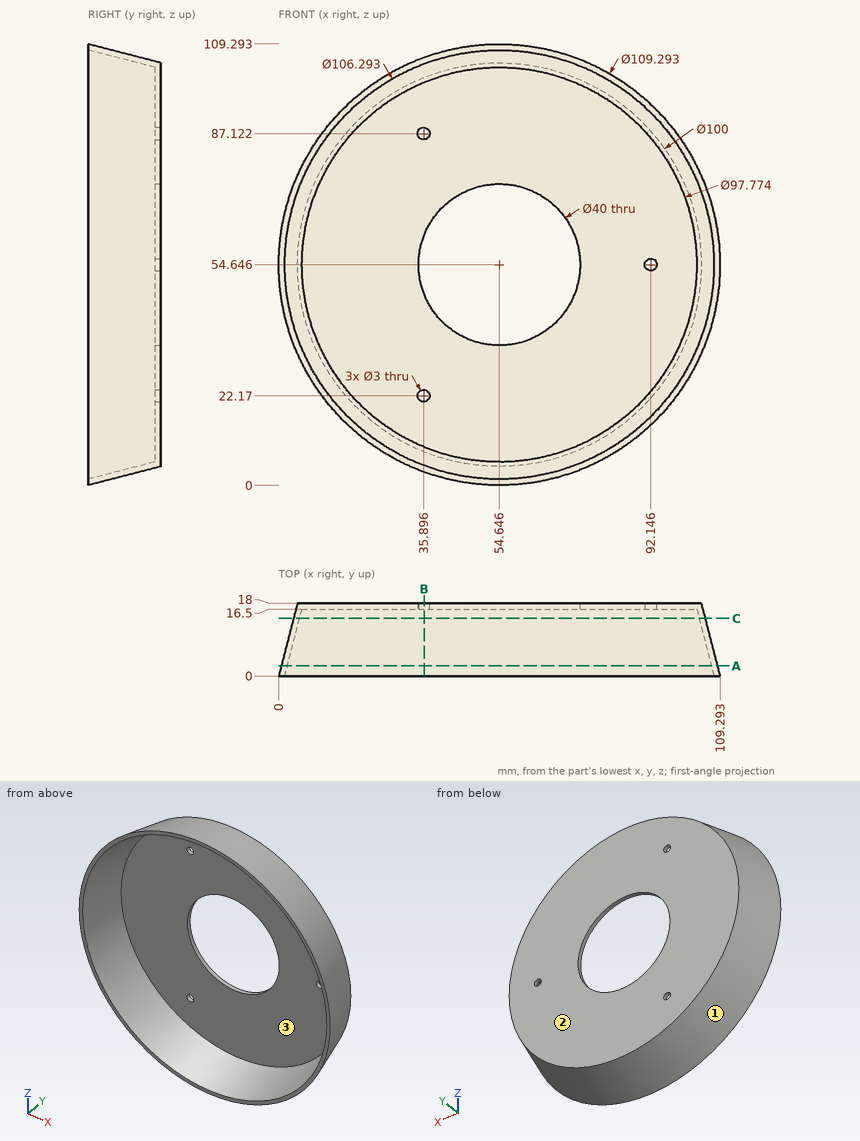
Can you work these out from the drawing? Everything is in mm from the part's minimum corner. Coordinates: 2 decimals unless noted, no trailing zeros. Loops run counter-clockwise (first coordinate to the right, second up) from the corner with the lowest first, then second, coordinate; pieces in that order, holes last.
1) Imagine slicing it at C-C (y = 14.25). List the corners of the cut face in (x, z) for me.
Reported:
outline: circle Ø101.94 at (54.65, 54.65); hole circle Ø98.94 at (54.65, 54.65)
2) Thinking about a two-plate mould opening in X: for the marked faces 1, 2 and 3, which applies, released by +X, released by -X, zero draft, split by the parting line, or undercut?
Reported:
face 1: split by the parting line
face 2: zero draft
face 3: undercut
3) Please list where these lines run through material, in increasing order: line 1 along Y through (x, z) = (29, 71.5); line 2 along X through (y, z) = (3.5, 43.5); line 3 along Z through (x, y) = (55, 8.75).
Reported:
line 1: y = 16.5 to 18
line 2: x = 2.07 to 3.61, 105.69 to 107.22
line 3: z = 2.26 to 3.76, 105.53 to 107.03
4) Will these pins go through, and if not, where does the flat tip stop? pin 1 Ø3.5 at (x, z) = (35.9, 87.12) entering from +Y; pin 2 Ø10 at (x, z) = (21, 45.5) entering from -Y; pin 3 Ø8 at (y, z) = (7.5, 45) entering from -X; pin 4 Ø8 at (y, z) = (8.5, 64) entering from +X.
Reported:
pin 1: stops at y = 18
pin 2: stops at y = 16.5
pin 3: stops at x = 1.59
pin 4: stops at x = 107.48
5) Imagine slicing it at A-A (y = 2.5). List the corners of the cut face in (x, z) for me (1 decimal).
Reported:
outline: circle Ø108 at (54.6, 54.6); hole circle Ø105 at (54.6, 54.6)
6) Imagine slicing it at B-B (x = 36). State how many separate pieces and enclosed holes the cut face has, and give its area (3 significant figures).
Reported:
separate pieces: 4
enclosed holes: 0
area: 162 mm2
